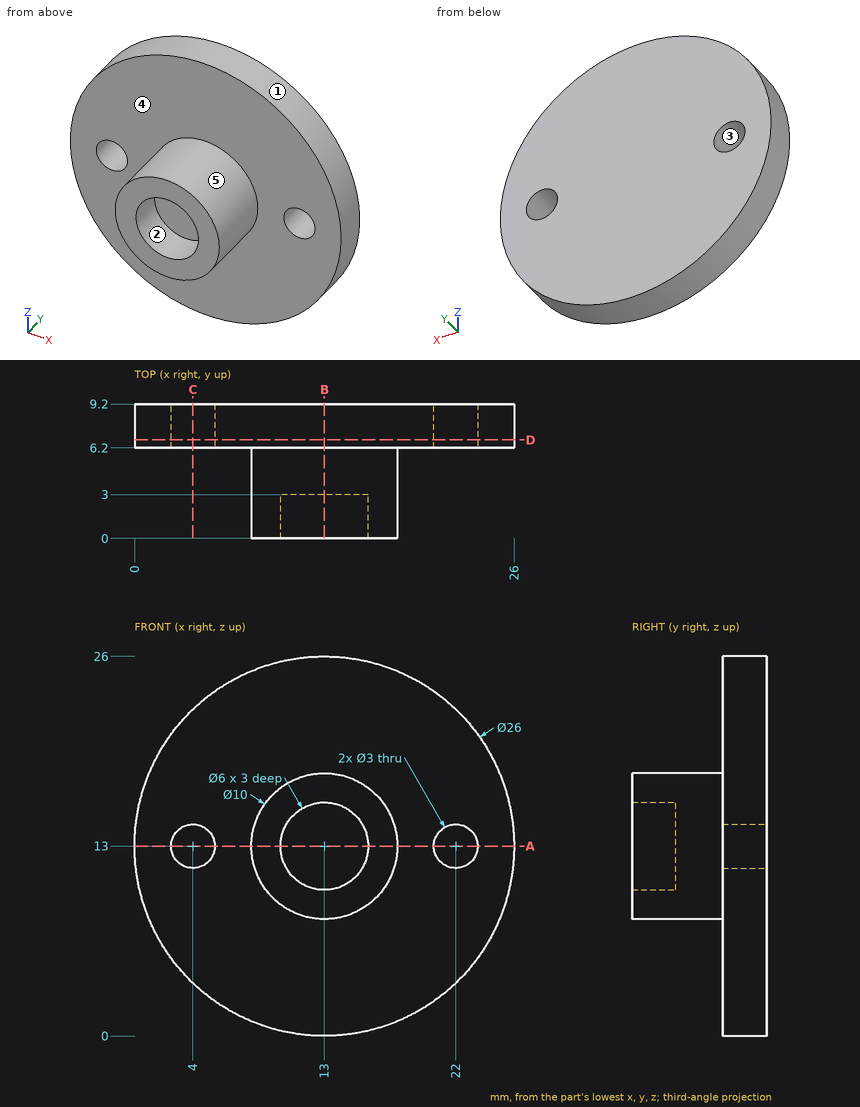
Design review of the part shown in the three views and the two pictorial views. Dimensions are in mm from the part's minimum x, y and z. A direction names the side the tool comes from. Round coordinates to 2 decimals unless told otherwise and drop trailing zeros. Loops run counter-clockwise (first coordinate to the right, second up) from the corner with the lowest first, then second, coordinate; pieces in that order, holes last. Notation, with made-up numbers: (35, 30.5) - (50, 30.5) arc R18 cw to (50, 64.5) - close; hole circle Ø11 at (72, -11). An arc over 180 degrees is marked (long way). Write each question's results on one line, items separated by ' | '. Start each with the question number.
Q1. Draft analysis for pull direction X (two halves, no side actions). For the marked faces 3, 4 and 5, state which applies: pulls with the +X half, pulls with the -X half, needs draft (parallel to the pull), parting line crosses it, or undercut.
Q2. Wall thickness on line 1 along X through (y, z) = (7.2, 13); line 2 along Z through (x, y) = (13, 0.8); line 3 along X through (y, z) = (7, 13.75): over which ranges is each line inside the solid? List them lowest first. Write a range as [from, to].
Q3. Take a section at A-A on z = 13. Give the boundary of the cut face in (x, y).
Q4. Take a section at C-C on x = 4. Give the boundary of the cut face in (y, z), plus the area to 3 significant figures.
Q5. Take a section at D-D on y = 6.75. Give the boundary of the cut face in (x, z).
Q6. Take a section at B-B on x = 13. Give the boundary of the cut face in (y, z), plus the area to 3 significant figures.
Q7. Insertion check: P1, Ø2.5, axis at x = 4, z = 13, coming from the +Y side; P2, Ø5, axis at x = 22, z = 13, coming from the -Y side; P3, Ø3, axis at x = 5.5, y = 7, coming from the -Z side; P4, Ø1.8, axis at x = 12, z = 12, coming from the -Y side. Each pin has a flat end and moves straight along its axis. Give the tip position at first contact, or say it passes through.
Q8. Tool access review of the marked faces 1 and 2: name each direction out of +Z, -Z, +X, -X, +Y, -Y from which nothing blocks a thin tool from reaching the whole face with its end or side.
Data:
1) face 3: undercut | face 4: needs draft | face 5: parting line crosses it
2) line 1: x = [0, 2.5], [5.5, 20.5], [23.5, 26] | line 2: z = [8, 10], [16, 18] | line 3: x = [0.02, 2.7], [5.3, 20.7], [23.3, 25.98]
3) outline: (0, 6.2) - (2.5, 6.2) - (2.5, 9.2) - (0, 9.2) - close; (5.5, 6.2) - (8, 6.2) - (8, 0) - (10, 0) - (10, 3) - (16, 3) - (16, 0) - (18, 0) - (18, 6.2) - (20.5, 6.2) - (20.5, 9.2) - (5.5, 9.2) - close; (23.5, 6.2) - (26, 6.2) - (26, 9.2) - (23.5, 9.2) - close
4) outline: (6.2, 3.62) - (9.2, 3.62) - (9.2, 11.5) - (6.2, 11.5) - close; (6.2, 14.5) - (9.2, 14.5) - (9.2, 22.38) - (6.2, 22.38) - close | area: 47.3 mm²
5) outline: circle Ø26 at (13, 13); hole circle Ø3 at (4, 13); hole circle Ø3 at (22, 13)
6) outline: (0, 8) - (6.2, 8) - (6.2, 0) - (9.2, 0) - (9.2, 26) - (6.2, 26) - (6.2, 18) - (0, 18) - (0, 16) - (3, 16) - (3, 10) - (0, 10) - close | area: 122 mm²
7) P1: passes through | P2: stops at y = 6.2 | P3: stops at z = 1.47 | P4: stops at y = 3
8) face 1: +Y, -Y | face 2: -Y
